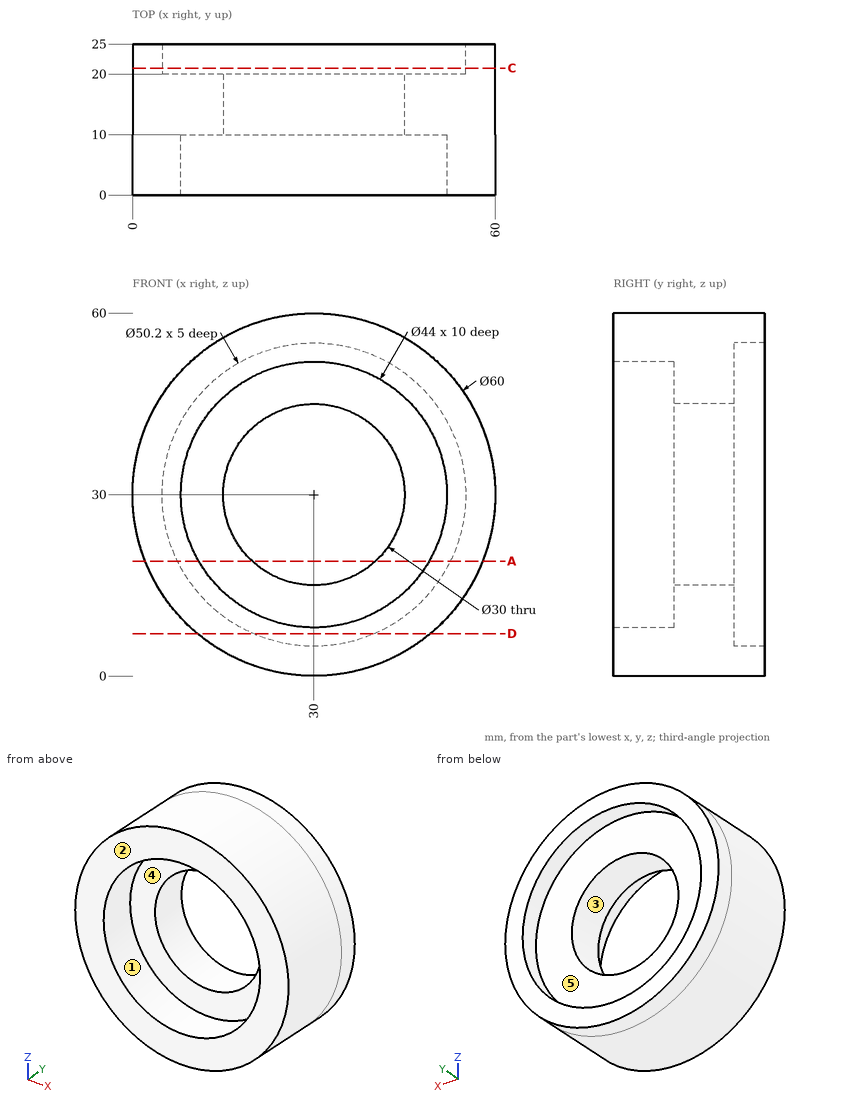
Print and shaded views of the part. All mm, measured from the part's lowest x, y and z. A direction names the side the tool comes from. Round coordinates to 2 decimals unless told otherwise and drop trailing zeros. Write each loop counter-clockwise with the first axis right and the second up, starting at its lowest first coordinate (ties: lowest second). Pieces come first, ordered by that corner, then holes. Notation, with made-up numbers: M 80,62.25 L 97,62.25 A35 cw 97,99.25 Z; hole C -26,-14 d5. An arc over 180 degrees is marked long. Use a Markdown table: item, result. Add a question column.
1. Drill centre lines: probe 1 along Z at (x, y) = (30, 16); probe 2 along Z at (x, y) = (30, 3); probe 3 along Y at (x, z) = (12.5, 36). Where is each one in solid material? Low to high.
2. Slice it at C-C on y = 21. Give the cut face in (x, z), then the cut area to 3 significant figures.
3. Slice it at D-D on z = 7. Give the cut face in (x, y), then the cut area to 3 significant figures.
4. Pull direction Z, two halves, no side cores. Call the marked faces 1 and 2: released by +Z, released by -Z, zero draft, split by the parting line, or undercut.
5. 3-axis set-ups, long thin cutter, end or side, ignore diameter. For the marked faces 3, 4 and 5: which of +Z, -Z, +X, -X, +Y, -Y reach the whole face in a straight line?
6. Slice it at A-A on z = 19. Give the cut face in (x, y).
7. Flat gauge pins, fed straight in: P1, Ø3, axis at x = 30, z = 47.5, coming from the +Y side; P2, Ø10, axis at y = 10.5, z = 14.5, coming from the -X side; P3, Ø6, axis at y = 12.5, z = 51, coming from the +X side; P4, Ø13, axis at x = 22.5, z = 27.5, coming from the -Y side. Where does each tip first touch, or does it go through?
Reply:
| question | item | result |
|---|---|---|
| 1 | probe 1 | z = 0 to 15, 45 to 60 |
| 1 | probe 2 | z = 0 to 8, 52 to 60 |
| 1 | probe 3 | y = 10 to 20 |
| 2 | outline | C 30,30 d60; hole C 30,30 d50.2 |
| 2 | area | 848 mm^2 |
| 3 | outline | M 10.74,0 L 49.26,0 L 49.26,25 L 40.05,25 L 40.05,20 L 19.95,20 L 19.95,25 L 10.74,25 Z |
| 3 | area | 863 mm^2 |
| 4 | face 1 | undercut |
| 4 | face 2 | zero draft |
| 5 | face 3 | +Y, -Y |
| 5 | face 4 | -Y |
| 5 | face 5 | +Y |
| 6 | outline | M 2.09,0 L 10.95,0 L 10.95,10 L 19.8,10 L 19.8,20 L 7.44,20 L 7.44,25 L 2.09,25 Z; M 40.2,10 L 49.05,10 L 49.05,0 L 57.91,0 L 57.91,25 L 52.56,25 L 52.56,20 L 40.2,20 Z |
| 7 | P1 | stops at y = 20 |
| 7 | P2 | stops at x = 1.9 |
| 7 | P3 | stops at x = 54 |
| 7 | P4 | passes through |
